from build123d import *

# Parameters (mm, degrees)
SKETCH4_W               = 25.4
SKETCH4_H               = 25.4
SKETCH4_W_2             = 22.225
SKETCH4_H_2             = 22.225
BOSS_EXTRUDE2_DEPTH     = 374.65
FILLET1_R               = 3.81
SKETCH5_R               = 3.2639
CUT_EXTRUDE1_DEPTH      = 1
CUT_EXTRUDE1_DEPTH_BACK = 26.4


with BuildPart() as part:
    # Sketch4 → Boss-Extrude2 (new body, symmetric)
    with BuildSketch(Plane.XY):
        Rectangle(SKETCH4_W, SKETCH4_H)
        Rectangle(SKETCH4_W_2, SKETCH4_H_2, mode=Mode.SUBTRACT)
    extrude(amount=BOSS_EXTRUDE2_DEPTH, both=True)

    # Fillet1
    fillet1_edges = [part.edges().sort_by_distance(p)[0] for p in [
        (12.7, -12.7, 0),
        (-12.7, -12.7, 0),
        (-12.7, 12.7, 0),
        (12.7, 12.7, 0),
    ]]
    fillet(fillet1_edges, radius=FILLET1_R)

    # Sketch5 → Cut-Extrude1 (cut, two sides)
    with BuildSketch(Plane(origin=(0, 12.7, 0), x_dir=(1, 0, 0), z_dir=(0, 1, 0))) as cut_extrude1_sk:
        with Locations((0, 127.59545203)):
            Circle(SKETCH5_R)
        with Locations((0, 266.10454797)):
            Circle(SKETCH5_R)
    extrude(amount=CUT_EXTRUDE1_DEPTH, mode=Mode.SUBTRACT)
    extrude(cut_extrude1_sk.sketch, amount=-CUT_EXTRUDE1_DEPTH_BACK, mode=Mode.SUBTRACT)


solid = part.part
The listing builds one solid part. Answer for the finished solid, in the listing's coordinates (mm). A direction names the side the tool comes from. Coordinates: 2 decimals unless noted, no trailing zeros. Loops run counter-clockwise (first coordinate to the right, second up) from the corner with the lowest first, then second, coordinate; pieces in that order, holes last. Notation, with made-up numbers: M -18,64.25 L -9,64.25 A22 ccw -9,84.25 Z; hole C -13,1.25 d5. An arc over 180 degrees is marked long. Answer in a Markdown table with one row per item.
1) Which of the six approach directions +Z, -Z, +X, -X, +Y, -Y give full straight-line access (tool end or side, diameter ignored) to faces 5 (the flat face through (0, -11.112, 5)), 6 (the flat face through (0, -12.7, 5))?
Answers below:
| item | result |
|---|---|
| face 5 | +Z, -Z |
| face 6 | +Z, -Z, +X, -X, -Y |
2) Find section A-A (y = -1). Determine the outline of the cut face in (x, z).
Answers below:
| item | result |
|---|---|
| outline | M -12.7,-374.65 L -11.11,-374.65 L -11.11,374.65 L -12.7,374.65 Z; M 11.11,-374.65 L 12.7,-374.65 L 12.7,374.65 L 11.11,374.65 Z |
3) Find the intervals of material crossed by probe 1 along Z at (x, y) = (0, 11.8); probe 2 along Y at (x, z) = (-4.25, -312.5), in increasing order.
Answers below:
| item | result |
|---|---|
| probe 1 | -374.65 to -269.37, -262.84 to -130.86, -124.33 to 374.65 |
| probe 2 | -12.7 to -11.11, 11.11 to 12.7 |
4) Determine the mould class of faces 1 (the flat face through (0, 12.7, 5)), 2 (the flat face through (12.7, 0, 5)), 3 (the flat face through (11.112, 0, 5)), 4 (the flat face through (-12.7, 0, 5)) for opening direction X: released by +X, released by -X, zero draft, split by the parting line, or undercut.
Answers below:
| item | result |
|---|---|
| face 1 | zero draft |
| face 2 | released by +X |
| face 3 | undercut |
| face 4 | released by -X |
5) Find section B-B (z = 194). Determine the outline of the cut face in (x, y), then the cut area to 3 significant figures.
Answers below:
| item | result |
|---|---|
| outline | M -12.7,-8.89 A3.81 ccw -8.89,-12.7 L 8.89,-12.7 A3.81 ccw 12.7,-8.89 L 12.7,8.89 A3.81 ccw 8.89,12.7 L -8.89,12.7 A3.81 ccw -12.7,8.89 Z; hole M -11.11,-11.11 L 11.11,-11.11 L 11.11,11.11 L -11.11,11.11 Z |
| area | 139 mm^2 |
